For this review, use the dimensioned drawing (mm, ordinates from the lowest corner) and the shaded views. A direction names the side the tool comes from. Give positions to 0.01 mm unless a question says otherwise; leave off trailing zeros. Loops run counter-clockwise (first coordinate to the right, second up) from the corner with the lowest first, then second, coordinate; pieces in that order, holes last. Notation, with made-up numbers: M 39,-25 L 44,-25 A13 cw 44,-21 Z; hole C 79,4 d5. An arc over 180 degrees is marked long. Use a Markdown table: item, result. Add a question column.
(1) Add section B-B, the plane y = 19. Give the boundary of the cut face in (x, z).
(2) Draft analysis for pull direction X (two halves, no side actions). For the marked faces 3, 4 and 5, state which applies: pulls with the +X half, pulls with the -X half, needs draft (parallel to the pull), parting line crosses it, or undercut.
(3) For probe 1 along X at (y, z) = (12, 6.25); probe 2 along Y at (x, z) = (3.5, 6.25); probe 3 along Y at (x, z) = (7.5, 5.5), list the stretches that pass through material, from the lowest coordinate up.
(4) Insertion check: pin 1 Ø0.7 at (y, z) = (32, 4.5) entering from +X; pin 2 Ø5 at (x, y) = (2, 5.5) entering from +Z; pin 3 Ø3 at (x, y) = (7.5, 17) entering from +Z (1 decimal). Each pin has a flat end and moves straight along its axis. Give the tip position at first contact, or say it passes through.
(5) Add section A-A, the plane z = 4.75. Give the boundary of the cut face in (x, y), then the cut area to 3 significant figures.
(6) For the marked faces 1 and 2, list the 3-axis set-ups (+Z, -Z, +X, -X, +Y, -Y) from which the entire face can be reached by the end or side of a thin tool; tool diameter is ignored.
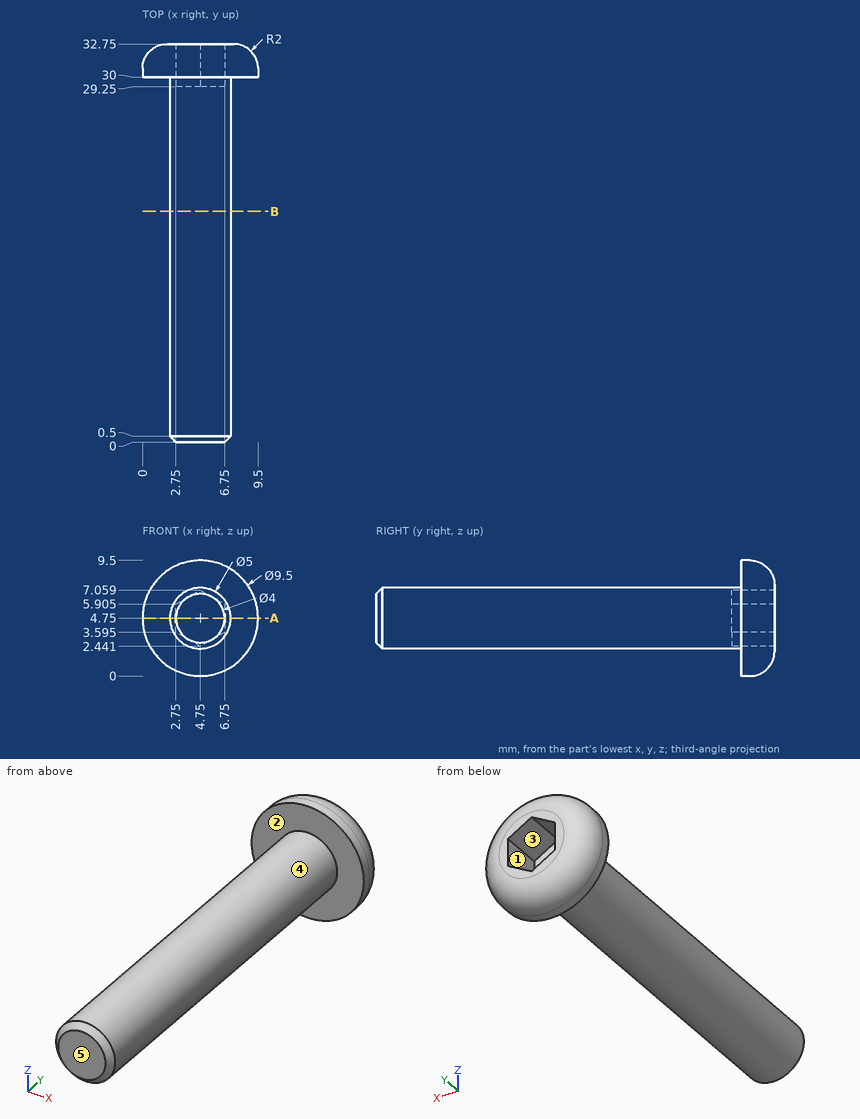
Established:
| question | item | result |
|---|---|---|
| 1 | outline | C 4.75,4.75 d5 |
| 2 | face 3 | undercut |
| 2 | face 4 | parting line crosses it |
| 2 | face 5 | needs draft |
| 3 | probe 1 | 2.75 to 6.75 |
| 3 | probe 2 | 0 to 29.25 |
| 3 | probe 3 | 30 to 32.75 |
| 4 | pin 1 | x = 9.28 |
| 4 | pin 2 | z = 7.24 |
| 4 | pin 3 | z = 6.9 |
| 5 | outline | M 0,30 L 2.25,30 L 2.25,0.5 L 2.75,0 L 6.75,0 L 7.25,0.5 L 7.25,30 L 9.5,30 L 9.5,30.75 A2 ccw 7.5,32.75 L 6.75,32.75 L 6.75,29.25 L 2.75,29.25 L 2.75,32.75 L 2,32.75 A2 ccw 0,30.75 Z |
| 5 | area | 160 mm^2 |
| 6 | face 1 | +Y |
| 6 | face 2 | -Y |
